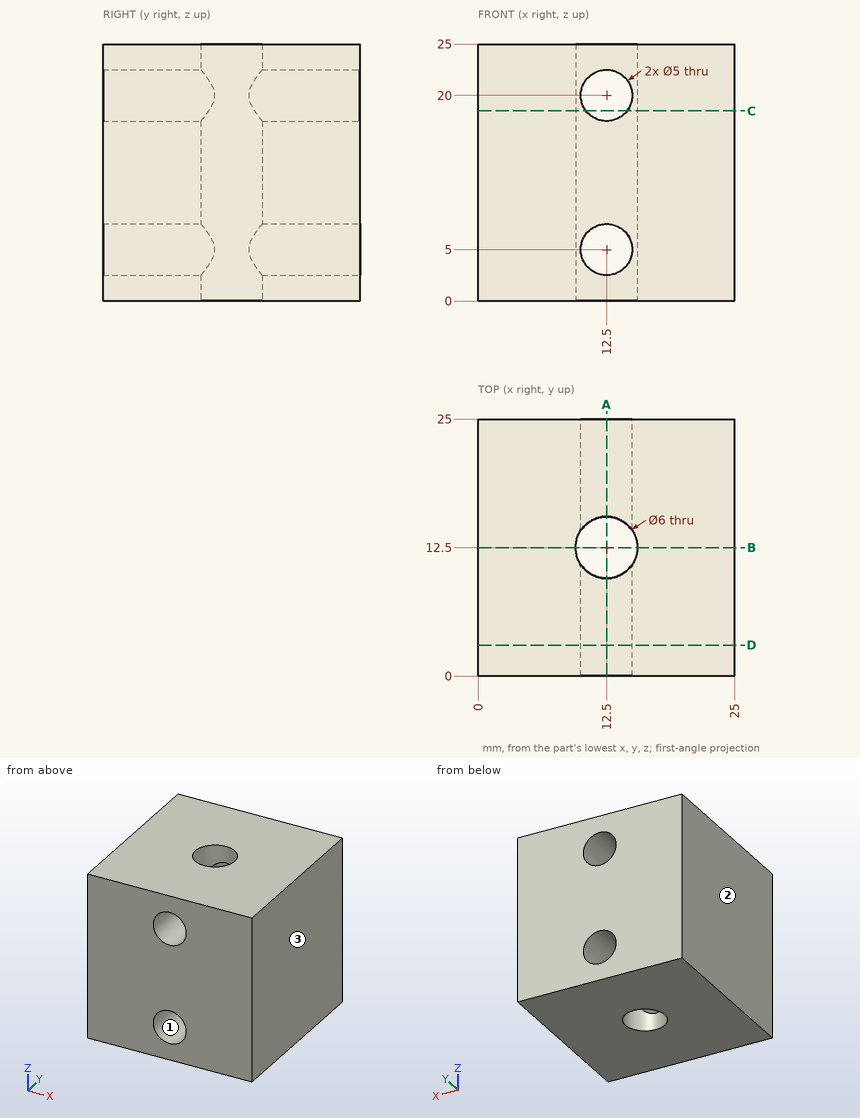
Can you work these out from the drawing? Everything is in mm from the part's minimum corner. Give positions to 0.01 mm unless a question says otherwise; leave off trailing zeros. Loops run counter-clockwise (first coordinate to the right, second up) from the corner with the lowest first, then second, coordinate; pieces in that order, holes last. Notation, with made-up numbers: (13, 52.25) -> (23, 52.25) arc R23 ccw to (23, 67.25) -> close; hole circle Ø9 at (63.25, 19.5). An arc over 180 degrees is marked (long way). Put each result on its own line as item: value.
(1) Thinking about a two-plate mould opening in X: for the marked faces 1, 2 and 3, which applies, pulls with the +X half, pulls with the -X half, needs draft (parallel to the pull), parting line crosses it, or undercut?
Computed:
face 1: undercut
face 2: pulls with the -X half
face 3: pulls with the +X half
(2) Imagine slicing it at D-D on y = 3. Write out the boundary of the cut face in (x, z), plus the area to 3 significant figures.
Computed:
outline: (0, 0) -> (25, 0) -> (25, 25) -> (0, 25) -> close; hole circle Ø5 at (12.5, 5); hole circle Ø5 at (12.5, 20)
area: 586 mm^2
(3) Imagine slicing it at C-C on z = 18.5. Write out the boundary of the cut face in (x, y).
Computed:
outline: (0, 0) -> (10.5, 0) -> (10.5, 10.26) arc R3 cw to (10.5, 14.74) -> (10.5, 25) -> (0, 25) -> close; (14.5, 0) -> (25, 0) -> (25, 25) -> (14.5, 25) -> (14.5, 14.74) arc R3 cw to (14.5, 10.26) -> close
(4) Imagine slicing it at B-B on y = 12.5. Write out the boundary of the cut face in (x, z), plus the area to 3 significant figures.
Computed:
outline: (0, 0) -> (9.5, 0) -> (9.5, 25) -> (0, 25) -> close; (15.5, 0) -> (25, 0) -> (25, 25) -> (15.5, 25) -> close
area: 475 mm^2
(5) Imagine slicing it at A-A on x = 12.5. Write out the boundary of the cut face in (y, z), plus the area to 3 significant figures.
Computed:
outline: (0, 0) -> (9.5, 0) -> (9.5, 2.5) -> (0, 2.5) -> close; (0, 7.5) -> (9.5, 7.5) -> (9.5, 17.5) -> (0, 17.5) -> close; (0, 22.5) -> (9.5, 22.5) -> (9.5, 25) -> (0, 25) -> close; (15.5, 0) -> (25, 0) -> (25, 2.5) -> (15.5, 2.5) -> close; (15.5, 7.5) -> (25, 7.5) -> (25, 17.5) -> (15.5, 17.5) -> close; (15.5, 22.5) -> (25, 22.5) -> (25, 25) -> (15.5, 25) -> close
area: 285 mm^2
(6) I'm going to push a flat-ended pin straight in: pin 1 Ø10 at (y, z) = (16.5, 16.5) entering from -X. Where does the tip first touch, or does it pass through?
Computed:
pin 1: x = 0
(7) Please list where these lines run through material, in increasing order: probe 1 along Z at (x, y) = (12.5, 4); probe 2 along Y at (x, z) = (14.25, 12.75); probe 3 along Y at (x, z) = (14.75, 24.25). Write a range as [from, to].
Computed:
probe 1: [0, 2.5], [7.5, 17.5], [22.5, 25]
probe 2: [0, 10.06], [14.94, 25]
probe 3: [0, 10.52], [14.48, 25]
